```python
from build123d import *

# Parameters (mm, degrees)
SKETCH1_W          = 152.4
SKETCH1_H          = 25.4
SHELL2_T           = -2.54
SKETCH2_R          = 12.7
CUT_EXTRUDE1_DEPTH = 218.017695131


with BuildPart() as part:
    # Sketch1 → Revolve1 (revolve)
    with BuildSketch(Plane.XY, mode=Mode.PRIVATE) as revolve1_sk:
        with Locations((76.2, 12.7)):
            Rectangle(SKETCH1_W, SKETCH1_H)
    revolve(revolve1_sk.sketch.rotate(Axis((0, 0, 0), (0, 1, 0)), 90), axis=Axis((0, 0, 0), (0, 1, 0)))

    # Shell2
    shell2_openings = [part.faces().sort_by_distance(p)[0] for p in [
        (0, 0, 0),
    ]]
    offset(amount=SHELL2_T, openings=shell2_openings, kind=Kind.INTERSECTION)

    # Sketch2 → Cut-Extrude1 (cut, through all)
    with BuildSketch(Plane(origin=(0, 25.4, 0), x_dir=(1, 0, 0), z_dir=(0, 1, 0))):
        with Locations(Location((0, 0, 0), (0, 0, 270))):
            Circle(SKETCH2_R)
    extrude(amount=-CUT_EXTRUDE1_DEPTH, mode=Mode.SUBTRACT)


solid = part.part
```
Design review of the part built by this model. Coordinates are the model's own, in mm. A direction names the side the tool comes from. Round coordinates to 2 decimals unless told otherwise and drop trailing zeros. Write each loop counter-clockwise with the first axis right and the second up, starting at its lowest first coordinate (ties: lowest second). Pieces come first, ordered by that corner, then holes. Notation, with made-up numbers: (71.5, -37) -> (87.5, -37) arc R28 ccw to (87.5, -1) -> close; hole circle Ø3 at (26, 71.25). An arc over 180 degrees is marked (long way). Answer in a Markdown table with one row per item.
Q1. Take a section at A-A, the plane z = 0. State the section outline as (x, y) points.
The answers:
| item | result |
|---|---|
| outline | (-152.4, 0) -> (-149.86, 0) -> (-149.86, 22.86) -> (-12.7, 22.86) -> (-12.7, 25.4) -> (-152.4, 25.4) -> close; (12.7, 22.86) -> (149.86, 22.86) -> (149.86, 0) -> (152.4, 0) -> (152.4, 25.4) -> (12.7, 25.4) -> close |
Q2. Take a section at D-D, the plane x = 42.5. State the section outline as (y, z) points.
The answers:
| item | result |
|---|---|
| outline | (0, -146.35) -> (25.4, -146.35) -> (25.4, 146.35) -> (0, 146.35) -> (0, 143.71) -> (22.86, 143.71) -> (22.86, -143.71) -> (0, -143.71) -> close |
Q3. Clearance check with flat-ended pins moving along their axes: pin 1 Ø5 at (x, z) = (111.5, -56) entering from -Y; pin 2 Ø10 at (y, z) = (12.5, -47) entering from +X; pin 3 Ø1.5 at (x, y) = (-22, 17) entering from +Z. State where each tip first meets the part, or that it passes through.
The answers:
| item | result |
|---|---|
| pin 1 | y = 22.86 |
| pin 2 | x = 146.5 |
| pin 3 | z = 150.91 |
Q4. Take a section at B-B, the plane x = 0. State the section outline as (y, z) points, then the cut area to 3 significant figures.
The answers:
| item | result |
|---|---|
| outline | (0, -152.4) -> (25.4, -152.4) -> (25.4, -12.7) -> (22.86, -12.7) -> (22.86, -149.86) -> (0, -149.86) -> close; (0, 149.86) -> (22.86, 149.86) -> (22.86, 12.7) -> (25.4, 12.7) -> (25.4, 152.4) -> (0, 152.4) -> close |
| area | 826 mm² |
Q5. Draft analysis for pull direction Z (two halves, no side actions). For faces 3 (the face through (146.296, 11.59, 32.487)), 4 (the face through (148.776, 12.878, 33.037)), 5 (the face through (101, 0, 112)), state which applies: +Z half, -Z half, draft (parallel to the pull), parting line (faces both ways), or undercut.
The answers:
| item | result |
|---|---|
| face 3 | undercut |
| face 4 | parting line |
| face 5 | draft |
Q6. For faces 1 (the face through (-2, 25.4, 32)), 2 (the face through (31, 22.86, -2)), list the 3-axis set-ups (+Z, -Z, +X, -X, +Y, -Y) from which the entire face can be reached by the end or side of a thin tool; tool diameter is ignored.
The answers:
| item | result |
|---|---|
| face 1 | +Z, -Z, +X, -X, +Y |
| face 2 | -Y |
Q7. Take a section at C-C, the plane y = 6.5. State the section outline as (x, z) points.
The answers:
| item | result |
|---|---|
| outline | circle Ø304.8 at (0, 0); hole circle Ø299.72 at (0, 0) |
Q8. To check wall thickness, follow L1, parallel to X at y = 24.45, z = 0; L2, parallel to Z at x = -2, y = 21; L3, parallel to X at y = 15, z = 0. State the ranges of each line that lie inside material, in increasing order. Write a range as [from, to].
The answers:
| item | result |
|---|---|
| L1 | [-152.4, -12.7], [12.7, 152.4] |
| L2 | [-152.39, -149.85], [149.85, 152.39] |
| L3 | [-152.4, -149.86], [149.86, 152.4] |
